Autodesk Inventor part; units mm, degrees
ref_plane "YZ Plane" through (0, 0, 0) normal (1, 0, 0) x (0, 1, 0)
ref_plane "XZ Plane" through (0, 0, 0) normal (0, 1, 0) x (-1, 0, 0)
ref_plane "XY Plane" through (0, 0, 0) normal (0, 0, 1) x (1, 0, 0)
sketch "Sketch1" plane through (0, 0, 0) normal (0, 0, 1) x (1, 0, 0)
  circle A0 centre (0, 0) radius 4
  dimension "Diameter" = 8
extrude "Extrusion1" add sketch "Sketch1" along normal blind 20.04
sketch "Sketch2" plane through (0, 0, 20.04) normal (0, 0, 1) x (1, 0, 0)
  circle A0 centre (0, 0) radius 4
extrude "Extrusion2" add sketch "Sketch2" along normal blind 4.96 draft 45
sketch "Sketch3" plane through (0, 0, 25) normal (0, 0, 1) x (1, 0, 0)
  circle A0 centre (0, 0) radius 8.96
  circle A1 centre (0, 0) radius 2.8868 construction
  line L0 (1.2084, 2.6217) -> (2.8746, 0.2644)
  line L1 (2.8746, 0.2644) -> (1.6662, -2.3573)
  line L2 (1.6662, -2.3573) -> (-1.2084, -2.6217)
  line L3 (-1.2084, -2.6217) -> (-2.8746, -0.2644)
  line L4 (-2.8746, -0.2644) -> (-1.6662, 2.3573)
  line L5 (-1.6662, 2.3573) -> (1.2084, 2.6217)
  dimension "Hex_Width" = 5
extrude "Extrusion3" cut sketch "Sketch3" against normal blind 3 contours L0 L1 L2 L3 L4 L5
thread "Thread1"
chamfer "Chamfer2" distance 0.8 angle 45 1 edges at (-4, 0, 0)
fillet "Fillet1" radius 0.1 1 edges at (-8.96, 0, 25)
equation "\"d10\" = Thread_Length"
equation "\"d13\" = Chamfer"
equation "\"Thread_Length\" = 20.04"
equation "\"Length\" = 25"
properties part number "SCREW, FLAT HD, P, 12.9, M8X1.25X25MM"
Geometry check sheet. Reference: the model listing, model coordinates, mm. A direction names the side the tool comes from. Give positions to 0.01 mm unless a question says otherwise; leave off trailing zeros. Loops run counter-clockwise (first coordinate to the right, second up) from the corner with the lowest first, then second, coordinate; pieces in that order, holes last. Notation, with made-up numbers: (-24, -7) -> (17, -7) arc R26 cw to (17, 7) -> close; hole circle Ø9 at (-5.5, 37). An arc over 180 degrees is marked (long way). Answer in a Markdown table with one row per item. Add a question column.
1) Cross-section at B-B on x = 0. Record the boundary of the cut face in (y, z), and give its area (3 significant figures).
2) Cross-section at A-A on z = 20.5. Record the boundary of the cut face in (x, y).
3) Material ranges on probe 1 along Z at (x, y) = (-0.25, -0.75); probe 2 along Z at (x, y) = (-6.5, 2.5); probe 3 along X at (y, z) = (1, 22.25), recorded low to high. Write a range as from..to.
4) Set-up check for faces 1 (the face through (-0.867, 3.905, 10.285)), 2 (the face through (0, 0, 0)), 3 (the face through (0, 0, 22)): record each of +Z, -Z, +X, -X, +Y, -Y from which the full face is reachable in a straight line by a thin tool's end or side.
5) Draft check along X on faces 4 (the face through (-0.93, -4.2, 20.34)), 5 (the face through (-2, -1.5, 23.5)), 6 (the face through (2, 2, 25)). Enter one of: pulls with the +X half, pulls with the -X half, needs draft (parallel to the pull), parting line crosses it, or undercut.
6) Gauge pin test, flat ends, axial feed: P1, Ø8, axis at x = -2.5, z = 19.5, coming from the -Y side; P2, Ø4, axis at x = 4.5, z = 15.5, coming from the -Y side; P3, Ø4, axis at y = -5, z = 13, coming from the +X side. Record the tip position at first contact, or that the pin passes through.
Outcome:
| question | item | result |
|---|---|---|
| 1 | outline | (-8.79, 24.83) -> (-4, 20.04) -> (-4, 0.8) -> (-3.2, 0) -> (3.2, 0) -> (4, 0.8) -> (4, 20.04) -> (8.79, 24.83) arc R0.1 ccw to (8.72, 25) -> (2.51, 25) -> (2.51, 22) -> (-2.51, 22) -> (-2.51, 25) -> (-8.72, 25) arc R0.1 ccw to start |
| 1 | area | 209 mm^2 |
| 2 | outline | circle Ø8.92 at (0, 0) |
| 3 | probe 1 | z = 0..22 |
| 3 | probe 2 | z = 23..25 |
| 3 | probe 3 | x = -6.13..-2.29, 2.35..6.13 |
| 4 | face 1 | -Z |
| 4 | face 2 | -Z, +X, -X, +Y, -Y |
| 4 | face 3 | +Z |
| 5 | face 4 | parting line crosses it |
| 5 | face 5 | undercut |
| 5 | face 6 | needs draft |
| 6 | P1 | stops at y = -7.18 |
| 6 | P2 | stops at y = -3.12 |
| 6 | P3 | stops at x = 2.65 |
